Autodesk Fusion 360 part; units mm, degrees
sketch "Sketch1" plane through (0, 0, 0) normal (0, 0, 1) x (1, 0, 0)
  line L0 (-0.9, 44.4476) -> (72, 44.4476)
  line L1 (72, 44.4476) -> (72, 2.6476)
  line L2 (72, 2.6476) -> (-0.9, 2.6476)
  line L3 (-0.9, 2.6476) -> (-0.9, 44.4476)
  line L4 (-0.9, 23.5476) -> (72, 23.5476) construction
  line L5 (72, 13.5476) -> (67, 13.5476)
  line L6 (67, 13.5476) -> (67, 33.5476)
  line L7 (67, 33.5476) -> (72, 33.5476)
  line L8 (72, 33.5476) -> (72, 13.5476)
  line L9 (-0.9, 28.5476) -> (-4.6, 28.5476)
  line L10 (-5.9, 27.2476) -> (-5.9, 19.8476)
  line L11 (-4.6, 18.5476) -> (-0.9, 18.5476)
  line L12 (-0.9, 18.5476) -> (-0.9, 28.5476)
  arc A0 (-4.6, 28.5476) -> (-5.9, 27.2476) centre (-4.6, 27.2476) ccw
  arc A1 (-5.9, 19.8476) -> (-4.6, 18.5476) centre (-4.6, 19.8476) ccw
  point P0 (-5.9, 28.5476)
  point P1 (-5.9, 18.5476)
  dimension "d1" = 72.9
  dimension "d2" = 41.8
  dimension "d5" = 20
  dimension "d6" = 5
  dimension "d7" = 10
  dimension "d8" = 5
  dimension "d9" = 1.3
extrude "Extrude1" add sketch "Sketch1" along normal blind 1 contours L0 L1 L2 L3 L5 L6 L7 L12 | L3 L9 L10 L11 L12 A0 A1
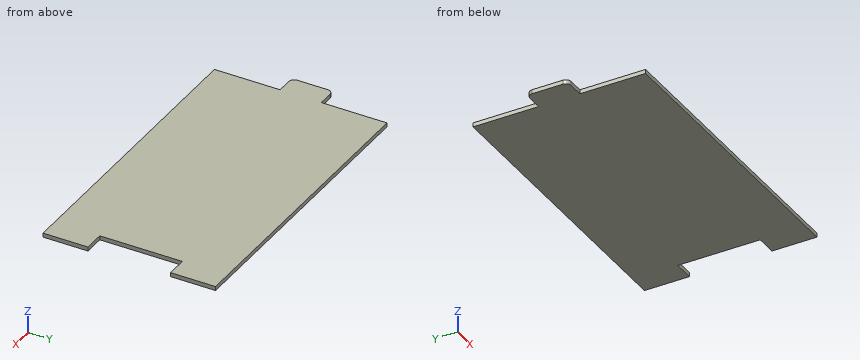
Geometry check sheet. Reference: the model listing, model coordinates, mm. Round coordinates to 2 decimals unless told otherwise and drop trailing zeros. Loops run counter-clockwise (first coordinate to the right, second up) from the corner with the lowest first, then second, coordinate; pieces in that order, holes last. Notation, with made-up numbers: M 21.5,84.5 L 46.5,84.5 A22 cw 46.5,103.5 Z; hole C -25.75,24 d8. An arc over 180 degrees is marked long. Return JSON: item names as keys, results as strings. Group by question number.
(1) Section check C-C, the plane y = 14.5. Enter the section's corners in (x, z), and give its area (3 significant figures).
(2) Scan lines: line 1 along X through (y, z) = (39, 0.35); line 2 along X through (y, z) = (23.5, 0.25); line 3 along Y through (x, z) = (69.5, 0.4). Record each from-to range of solid material in increasing order. Write a range as [from, to].
(3) Go/stop test with flat-tipped pins: pin 1 (0.5 mm diameter, centred on x = -2.5, z = 0.5, fed in from -Y); pin 2 (0.5 mm diameter, centred on y = 26, z = 0.5, fed in from +X); pin 3 (0.5 mm diameter, centred on y = 33, z = 0.5, fed in from -X). Record where each tip stops, or that it passes through.
(4) Section check B-B, the plane y = 35. Enter the section's corners in (x, z).
(5) Section check A-A, the plane z = 0.25. Enter the section's corners in (x, y).
Data:
{
 "1": {"outline": "M -0.9,0 L 67,0 L 67,1 L -0.9,1 Z", "area": "67.9 mm²"},
 "2": {"line 1": "[-0.9, 72]", "line 2": "[-5.9, 67]", "line 3": "[2.65, 13.55], [33.55, 44.45]"},
 "3": {"pin 1": "y = 18.55", "pin 2": "x = 67", "pin 3": "x = -0.9"},
 "4": {"outline": "M -0.9,0 L 72,0 L 72,1 L -0.9,1 Z"},
 "5": {"outline": "M -5.9,19.85 A1.3 ccw -4.6,18.55 L -0.9,18.55 L -0.9,2.65 L 72,2.65 L 72,13.55 L 67,13.55 L 67,33.55 L 72,33.55 L 72,44.45 L -0.9,44.45 L -0.9,28.55 L -4.6,28.55 A1.3 ccw -5.9,27.25 Z"}
}
